Verification items for the finished model (mm, model axes). Coordinates: 2 decimals unless noted, no trailing zeros. Loops run counter-clockwise (first coordinate to the right, second up) from the corner with the lowest first, then second, coordinate; pieces in that order, holes last. Notation, with made-up numbers: (-2.75, -5) - (9.25, -5) arc R18 ccw to (9.25, 10) - close; hole circle Ø2 at (45, 13.25). An arc over 180 degrees is marked (long way). One line per item, written item: value. Start each with the question number.
(1) Thickness scan on probe 1 along Y at (x, z) = (-0.15, 8); probe 2 along X at (y, z) = (-0.95, 8.25). Record the ranges inside material, lowest first. Write a range as [from, to].
(2) Section check D-D (z = 1.5). Record the boundary of the cut face in (x, y).
(3) Draft check along X on faces 1 (the face through (0, 0, 0)), 2 (the face through (-3, 0, 5)), 3 (the face through (0, -1.25, 8)). Enter one of: +X half, -X half, draft (parallel to the pull), parting line (faces both ways), or undercut.
(4) Section check A-A (z = 7.75). Record the boundary of the cut face in (x, y), plus the area to 3 significant figures.
(5) Section check B-B (x = 0). Record the boundary of the cut face in (y, z), plus the area to 3 significant figures.
(6) Gauge pin test, flat end, axial feed: P1, Ø1, axis at y = 2, z = 7, coming from the +X side. Record the tip position at first contact, or that the pin passes through.
```python
from build123d import *

# Parameters (mm, degrees)
SKETCH_R     = 3
PAD_DEPTH    = 10
SKETCH001_W  = 2.5
SKETCH001_H  = 2.5
POCKET_DEPTH = 4
FILLET_R     = 0.5


with BuildPart() as part:
    # Sketch → Pad (new body)
    with BuildSketch(Plane.XY):
        Circle(SKETCH_R)
    extrude(amount=PAD_DEPTH)

    # Sketch001 (on Face3 of Pad) → Pocket (cut)
    with BuildSketch(Plane.XY.offset(10)):
        Rectangle(SKETCH001_W, SKETCH001_H)
    extrude(amount=-POCKET_DEPTH, mode=Mode.SUBTRACT)

    # Fillet
    fillet_edges = [part.edges().sort_by_distance(p)[0] for p in [
        (-3, 0, 0),
    ]]
    fillet(fillet_edges, radius=FILLET_R)


solid = part.part
```
Responses:
1. probe 1: y = [-3, -1.25], [1.25, 3]
1. probe 2: x = [-2.85, -1.25], [1.25, 2.85]
2. outline: circle Ø6 at (0, 0)
3. face 1: draft
3. face 2: parting line
3. face 3: undercut
4. outline: circle Ø6 at (0, 0); hole (-1.25, -1.25) - (1.25, -1.25) - (1.25, 1.25) - (-1.25, 1.25) - close
4. area: 22.0 mm²
5. outline: (-3, 0.5) arc R0.5 ccw to (-2.5, 0) - (2.5, 0) arc R0.5 ccw to (3, 0.5) - (3, 10) - (1.25, 10) - (1.25, 6) - (-1.25, 6) - (-1.25, 10) - (-3, 10) - close
5. area: 49.9 mm²
6. P1: stops at x = 2.6
